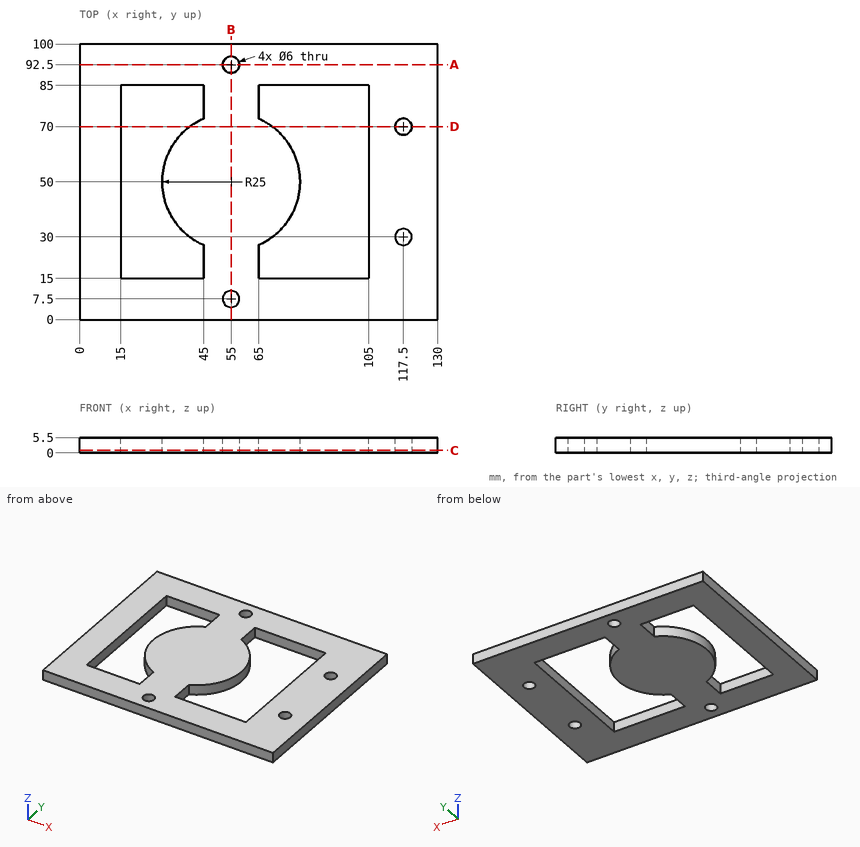
Check sheet for the drawn part. Datum: minimum x, y, z corner. Units: mm. Round coordinates to 2 decimals unless told otherwise and drop trailing zeros. Loops run counter-clockwise (first coordinate to the right, second up) from the corner with the lowest first, then second, coordinate; pieces in that order, holes last. Notation, with made-up numbers: (-5, 10.5) -> (9, 10.5) arc R21 ccw to (9, 45.5) -> close; hole circle Ø2 at (28, 38). An arc over 180 degrees is marked (long way). Put each result on its own line as item: value. Start each with the question number.
1. Section check B-B (x = 55). Enter the section's corners in (y, z), plus the area to 3 significant figures.
2. Section check C-C (z = 0.9). Enter the section's corners in (x, y), plus the area to 3 significant figures.
3. Section check A-A (y = 92.5). Enter the section's corners in (x, z), plus the area to 3 significant figures.
4. Section check D-D (y = 70). Enter the section's corners in (x, z).
5. Scan lines: probe 1 along X at (y, z) = (84.5, 3.3); probe 2 along Y at (x, z) = (117.5, 1.4); probe 3 along Y at (x, z) = (55, 3.4). Record each from-to range of solid material in increasing order.
Findings:
1. outline: (0, 0) -> (4.5, 0) -> (4.5, 5.5) -> (0, 5.5) -> close; (10.5, 0) -> (89.5, 0) -> (89.5, 5.5) -> (10.5, 5.5) -> close; (95.5, 0) -> (100, 0) -> (100, 5.5) -> (95.5, 5.5) -> close
1. area: 484 mm^2
2. outline: (0, 0) -> (130, 0) -> (130, 100) -> (0, 100) -> close; hole (15, 15) -> (45, 15) -> (45, 27.09) arc R25 cw to (45, 72.91) -> (45, 85) -> (15, 85) -> close; hole circle Ø6 at (55, 7.5); hole circle Ø6 at (55, 92.5); hole (65, 15) -> (105, 15) -> (105, 85) -> (65, 85) -> (65, 72.91) arc R25 cw to (65, 27.09) -> close; hole circle Ø6 at (117.5, 30); hole circle Ø6 at (117.5, 70)
2. area: 8,980 mm^2
3. outline: (0, 0) -> (52, 0) -> (52, 5.5) -> (0, 5.5) -> close; (58, 0) -> (130, 0) -> (130, 5.5) -> (58, 5.5) -> close
3. area: 682 mm^2
4. outline: (0, 0) -> (15, 0) -> (15, 5.5) -> (0, 5.5) -> close; (40, 0) -> (70, 0) -> (70, 5.5) -> (40, 5.5) -> close; (105, 0) -> (114.5, 0) -> (114.5, 5.5) -> (105, 5.5) -> close; (120.5, 0) -> (130, 0) -> (130, 5.5) -> (120.5, 5.5) -> close
5. probe 1: x = 0 to 15, 45 to 65, 105 to 130
5. probe 2: y = 0 to 27, 33 to 67, 73 to 100
5. probe 3: y = 0 to 4.5, 10.5 to 89.5, 95.5 to 100
